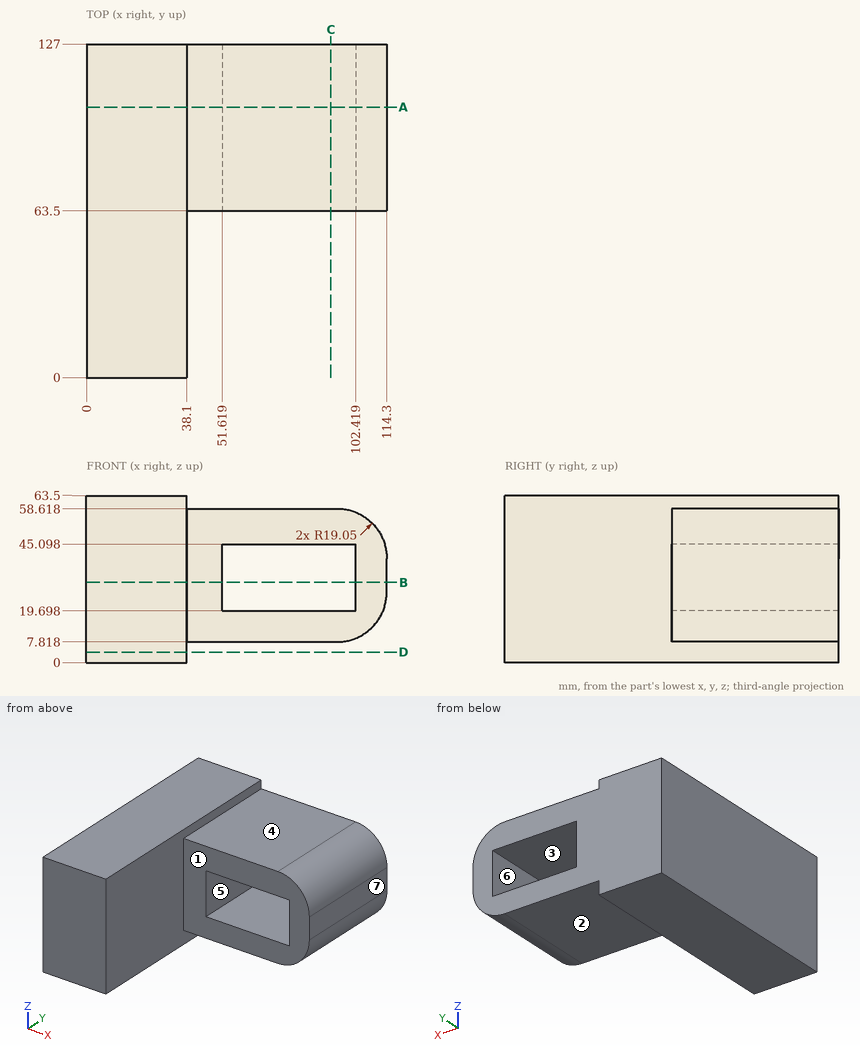
Job drawing, mm, ordinate dimensions from the low corner. One solid piece. A direction names the side the tool comes from. Coordinates: 2 decimals unless noted, no trailing zeros. Loops run counter-clockwise (first coordinate to the right, second up) from the corner with the lowest first, then second, coordinate; pieces in that order, holes last. Notation, with made-up numbers: (-7, -17.5) - (28, -17.5) arc R33 ccw to (28, 10.5) - close; hole circle Ø9 at (-4, -20). An arc over 180 degrees is marked (long way). Answer as a JSON object with one key per item and string values. Group by question number.
(1) Cut at C-C (x = 93). Give the cut face in (y, z).
(2) Flat gauge pins, fed straight in: pin 1 (8 mm diameter, centred on x = 101.5, y = 85.5, fed in from +Z); pin 2 (6 mm diameter, centred on x = 101.5, z = 8, fed in from -Y); pin 3 (17 mm diameter, centred on x = 69.5, y = 97, fed in from +Z). Where does each tip first touch, or does it go through?
(3) Two-plate mould, pull along X, no slides. Class the marked faces 4, 5, 6 and 7: released by +X, released by -X, zero draft, split by the parting line, or undercut.
(4) Tool access for the marked faces 1, 2 and 3: list every direction of +Z, -Z, +X, -X, +Y, -Y with a clear straight run to the whole face (end or side of a thin tool).
(5) Cut at A-A (y = 103). Give the cut face in (x, z), then the cut area to 3 significant figures.
(6) Probe line 1 along Z through (x, y) = (61.5, 107); line 2 along Y through (x, z) = (85.5, 50); line 3 along X through (y, z) = (26.5, 32). List the from-to ranges inside material, lowest first.
(7) Cut at B-B (z = 30.5). Give the cut face in (x, y), then the cut area to 3 significant figures.
(8) Cut at D-D (z = 4). Give the cut face in (x, y).
Geometry says:
{
 "1": {"outline": "(63.5, 7.82) - (127, 7.82) - (127, 19.7) - (63.5, 19.7) - close; (63.5, 45.1) - (127, 45.1) - (127, 58.62) - (63.5, 58.62) - close"},
 "2": {"pin 1": "stops at z = 58.48", "pin 2": "stops at y = 63.5", "pin 3": "stops at z = 58.62"},
 "3": {"face 4": "zero draft", "face 5": "undercut", "face 6": "undercut", "face 7": "released by +X"},
 "4": {"face 1": "+Z, -Z, +X, -Y", "face 2": "-Z, +X, +Y, -Y", "face 3": "+Y, -Y"},
 "5": {"outline": "(0, 0) - (38.1, 0) - (38.1, 7.82) - (95.25, 7.82) arc R19.05 ccw to (114.3, 26.87) - (114.3, 39.57) arc R19.05 ccw to (95.25, 58.62) - (38.1, 58.62) - (38.1, 63.5) - (0, 63.5) - close; hole (51.62, 19.7) - (102.42, 19.7) - (102.42, 45.1) - (51.62, 45.1) - close", "area": "4,840 mm^2"},
 "6": {"line 1": "z = 7.82 to 19.7, 45.1 to 58.62", "line 2": "y = 63.5 to 127", "line 3": "x = 0 to 38.1"},
 "7": {"outline": "(0, 0) - (38.1, 0) - (38.1, 63.5) - (51.62, 63.5) - (51.62, 127) - (0, 127) - close; (102.42, 63.5) - (114.3, 63.5) - (114.3, 127) - (102.42, 127) - close", "area": "6,450 mm^2"},
 "8": {"outline": "(0, 0) - (38.1, 0) - (38.1, 127) - (0, 127) - close"}
}
